Geometry check sheet. Reference: the model listing, model coordinates, mm. A direction names the side the tool comes from. Round coordinates to 2 decimals unless told otherwise and drop trailing zeros. Write each loop counter-clockwise with the first axis right and the second up, starting at its lowest first coordinate (ties: lowest second). Pieces come first, ordered by that corner, then holes. Notation, with made-up numbers: (85.5, 73.5) -> (134.5, 73.5) arc R17 cw to (134.5, 80.5) -> close; hole circle Ø7 at (43.25, 74). An arc over 180 degrees is marked (long way). One line per question, with ' | ' between items.
```python
from build123d import *
from build123d.topology import SkipClean

# Parameters (mm, degrees)
SKETCH1_R                   = 6
EXTRUDE1_DEPTH              = 10
SKETCH2_R                   = 13.25
CUT_EXTRUDE1_DEPTH          = 6
SKETCH3_R                   = 1.6
CUT_EXTRUDE2_DEPTH          = 10
SKETCH4_W                   = 7
SKETCH4_H                   = 10
SKETCH4_R                   = 1.6
EXTRUDE3_DEPTH              = 9
FILLET2_R                   = 5
CHAMFER4_SIZE               = 6
CHAMFER4_SIZE2              = 10.392304845
M4_TAPPED_HOLE1_D           = 3.3
M4_TAPPED_HOLE1_DEPTH       = 10.1
M4_TAPPED_HOLE1_TIP         = 0.991420021
SKETCH6_R                   = 1.25
EXTRUDE4_DEPTH              = 4
M3_START                    = 12.4999999
M3_TAPPED_HOLE1_OUTLINE_R   = 1.25
M3_TAPPED_HOLE1_DEPTH       = 0.5000001
M3_START_2                  = -13
M3_TAPPED_HOLE1_2_OUTLINE_R = 1.25
M3_TAPPED_HOLE1_2_DEPTH     = 0.4999999
EXTRUDE5_REACH              = 37.285
SKETCH8_W                   = 6
SKETCH8_H                   = 4.052940251


with BuildPart() as part:
    # Sketch1 → Extrude1 (new body)
    with BuildSketch(Plane.XY):
        Polygon((-17, 0), (-28, 0), (-28, -10), (28, -10), (28, 0), (17, 0), (17, 18), (-17, 18), align=None)
        with Locations((0, 6.53e-07)):
            Circle(SKETCH1_R, mode=Mode.SUBTRACT)
    extrude(amount=EXTRUDE1_DEPTH)

    # Sketch2 → Cut-Extrude1 (cut)
    with BuildSketch(Plane(origin=(0, 0, 0), x_dir=(-1, 0, 0), z_dir=(0, 0, -1))):
        Circle(SKETCH2_R)
    extrude(amount=-CUT_EXTRUDE1_DEPTH, mode=Mode.SUBTRACT)

    # Sketch3 → Cut-Extrude2 (cut)
    with BuildSketch(Plane(origin=(0, 0, 0), x_dir=(-1, 0, 0), z_dir=(0, 1, 0))):
        with Locations(Location((-24.5, 5, 0), (0, 0, 90))):
            Circle(SKETCH3_R)
        with Locations(Location((24.5, 5, 0), (0, 0, 90))):
            Circle(SKETCH3_R)
    extrude(amount=-CUT_EXTRUDE2_DEPTH, mode=Mode.SUBTRACT)

    # Sketch4 → Extrude3 (add)
    # profile 1 of 2: a face of its own
    with SkipClean():  # the faces are left unmerged after this step: merging them gives an invalid solid
        with BuildSketch(Plane.XZ.offset(10)):
            with Locations((-24.5, 5)):
                Rectangle(SKETCH4_W, SKETCH4_H)
            with Locations((-24.5, 5)):
                Circle(SKETCH4_R, mode=Mode.SUBTRACT)
        # profile 2 of 2: a face of its own
        with BuildSketch(Plane.XZ.offset(10)):
            with Locations((24.5, 5)):
                Rectangle(SKETCH4_W, SKETCH4_H)
            with Locations((24.5, 5)):
                Circle(SKETCH4_R, mode=Mode.SUBTRACT)
        extrude(amount=EXTRUDE3_DEPTH)
    add(part.part.scale(1), mode=Mode.REPLACE)  # the faces are merged on a copy

    # Fillet2
    fillet2_edges = [part.edges().sort_by_distance(p)[0] for p in [
        (28, -5, 0),
        (28, -5, 10),
        (-28, -9.5, 0),
        (-28, -9.5, 10),
    ]]
    fillet(fillet2_edges, radius=FILLET2_R - 0.0001)  # a hair under: the kernel refuses the full size

    # Chamfer4
    chamfer4_edges = [part.edges().sort_by_distance(p)[0] for p in [
        (0, 18, 10),
    ]]
    chamfer4_side = [part.faces().sort_by_distance(p)[0] for p in [
        (0, 18, 5),
    ]]
    chamfer(chamfer4_edges, length=CHAMFER4_SIZE, length2=CHAMFER4_SIZE2, reference=chamfer4_side[0])

    # M4 Tapped Hole1
    with Locations(Plane(origin=(-24.5, -19, 5), x_dir=(0, 0, -1), z_dir=(0, -1, 0))):
        with Locations((0, 0), (0, 49)):
            Hole(M4_TAPPED_HOLE1_D / 2, depth=M4_TAPPED_HOLE1_DEPTH)
            with Locations((0, 0, -(M4_TAPPED_HOLE1_DEPTH + M4_TAPPED_HOLE1_TIP / 2))):  # 118° drill point
                Cone(0, M4_TAPPED_HOLE1_D / 2, M4_TAPPED_HOLE1_TIP, mode=Mode.SUBTRACT)

    # Sketch6 → Extrude4 (cut)
    with BuildSketch(Plane.ZY.offset(17)):
        with Locations((3.33604719, 14.15)):
            Circle(SKETCH6_R)
        with Locations((6.332495088, 8.96)):
            Circle(SKETCH6_R)
    extrude4 = extrude(amount=-EXTRUDE4_DEPTH, mode=Mode.SUBTRACT)

    # Mirror1: Extrude4 across plane
    add(extrude4.mirror(Plane(origin=(0, 0, 0), x_dir=(0, 0, 1), z_dir=(1, 0, 0))), mode=Mode.SUBTRACT)

    # M3 Tapped Hole1: read off the stored shape, not the designer's step
    # M3 Tapped Hole1 outline → M3 Tapped Hole1 (cut)
    with BuildSketch(Plane.YZ.offset(M3_START)):
        with Locations((14.15, 3.33604719)):
            Circle(M3_TAPPED_HOLE1_OUTLINE_R)
        with Locations((8.96, 6.332495088)):
            Circle(M3_TAPPED_HOLE1_OUTLINE_R)
    extrude(amount=M3_TAPPED_HOLE1_DEPTH, mode=Mode.SUBTRACT)

    # M3 Tapped Hole1 2 outline → M3 Tapped Hole1 2 (cut)
    with BuildSketch(Plane.YZ.offset(M3_START_2)):
        with Locations((14.15, 3.33604719)):
            Circle(M3_TAPPED_HOLE1_2_OUTLINE_R)
        with Locations((8.96, 6.332495088)):
            Circle(M3_TAPPED_HOLE1_2_OUTLINE_R)
    extrude(amount=M3_TAPPED_HOLE1_2_DEPTH, mode=Mode.SUBTRACT)

    # M3 Tapped Hole1 3 outline → M3 Tapped Hole1 3 (revolve, cut)
    with BuildSketch(Plane(origin=(0, 14.15, 3.33604719), x_dir=(0, 1, 0), z_dir=(0, 0, -1))):
        Polygon((0, 12.5), (0, 11.748924226), (1.25, 12.5), align=None)
        Polygon((1.25, -12.5), (0, -11.748924226), (0, -12.5000001), align=None)
    revolve(axis=Axis((0, 14.15, 3.33604719), (1, 0, 0)), mode=Mode.SUBTRACT)

    # M3 Tapped Hole1 4 outline → M3 Tapped Hole1 4 (revolve, cut)
    with BuildSketch(Plane(origin=(0, 8.96, 6.332495088), x_dir=(0, 1, 0), z_dir=(0, 0, -1))):
        Polygon((0, 12.5), (0, 11.748924226), (1.25, 12.5), align=None)
        Polygon((1.25, -12.5), (0, -11.748924226), (0, -12.5000001), align=None)
    revolve(axis=Axis((0, 8.96, 6.332495088), (1, 0, 0)), mode=Mode.SUBTRACT)

    # Extrude5: up to this face of the body (flat: up to its plane)
    extrude5_end = Plane(part.part.faces().sort_by_distance((-16.468587934, 3.803847577, 10))[0])
    # Sketch8 → Extrude5 (cut, up to the picked face)
    with BuildSketch(Plane(origin=(0, 0, 0), x_dir=(-1, 0, 0), z_dir=(0, 0, -1)), mode=Mode.PRIVATE) as extrude5_sk1:
        with Locations((0, 13.973529875)):
            Rectangle(SKETCH8_W, SKETCH8_H)
    extrude5_tool1 = split(extrude(extrude5_sk1.sketch, amount=-EXTRUDE5_REACH, mode=Mode.PRIVATE), bisect_by=extrude5_end, keep=Keep.BOTH, mode=Mode.PRIVATE)
    add(extrude5_tool1.solids().sort_by(Axis((0, 13.97353, 0), (0, 0, 1)))[0], mode=Mode.SUBTRACT)


solid = part.part
```
(1) Sectioned sample at B-B on x = 0. Record the cut outline in (y, z).
Resolved:
outline: (-10, 6) -> (-6, 6) -> (-6, 10) -> (-10, 10) -> close; (6, 6) -> (11.95, 6) -> (11.95, 7.49) -> (7.61, 10) -> (6, 10) -> close; (16, 0) -> (18, 0) -> (18, 4) -> (16, 5.15) -> close
(2) Sectioned sample at D-D on x = -24.5. Record the cut outline in (y, z), then the cut area to 3 significant figures.
Resolved:
outline: (-19, 0.23) -> (0, 0.23) -> (0, 3.4) -> (-8.87, 3.4) -> (-8.9, 3.35) -> (-19, 3.35) -> close; (-19, 6.65) -> (-8.9, 6.65) -> (-8.87, 6.6) -> (0, 6.6) -> (0, 9.77) -> (-19, 9.77) -> close | area: 119 mm2
(3) Sectioned sample at A-A on y = -16.5. Count the separate pieces of the cut face and the enclosed holes in it, then the cut area to 3 significant figures.
Resolved:
separate pieces: 2 | enclosed holes: 2 | area: 101 mm2
(4) Go/stop test with flat-tipped pins: pin 1 (3 mm diameter, centred on x = -23, z = 2.5, fed in from +Y); pin 2 (4.5 mm diameter, centred on y = 13.5, z = 2, fed in from -X); pin 3 (3 mm diameter, centred on y = 14, z = 6.5, fed in from +X). Record where each tip stops, or that it passes through.
Resolved:
pin 1: stops at y = 0 | pin 2: stops at x = -17 | pin 3: stops at x = 17
(5) Access from +Z, -Z, +X, -X, +Y, -Y to the whole of each face (thin tool, end or side, straight path). Record for faces 4 (the flat face through (0, -10, 7)), 5 (the flat face through (-3, 14, 3)), 6 (the cylindrical face through (14.78, 9.43, 7.49)), 7 (the flat face through (21, 0, 5)), 8 (the cylindrical face through (26.136, -13.879, 4.785)).
Resolved:
face 4: +Z, -Z, -Y | face 5: +Z, -Z | face 6: +X | face 7: +Z, -Z, +X, +Y | face 8: -Y
(6) Material ranges on line 1 (X direction, y = -15, z = 5); line 2 (X direction, y = 13, z = 5.5); line 3 (X direction, y = -12.5, z = 3.5), recorded low to high.
Resolved:
line 1: x = -28 to -26.15, -22.85 to -21, 21 to 22.85, 26.15 to 28 | line 2: x = -17 to -3, 3 to 17 | line 3: x = -27.77 to -25.19, -23.81 to -21, 21 to 23.81, 25.19 to 27.77
(7) Draft check along Y on faces 1 (the flat face through (0, 16, 3)), 2 (the conical face through (11.879, 9.077, 6.516)), 3 (the flat face through (-4, 13, 0)). Enter one of: +Y half, -Y half, draft (parallel to the pull), parting line (faces both ways), or undercut.
Resolved:
face 1: -Y half | face 2: undercut | face 3: draft
